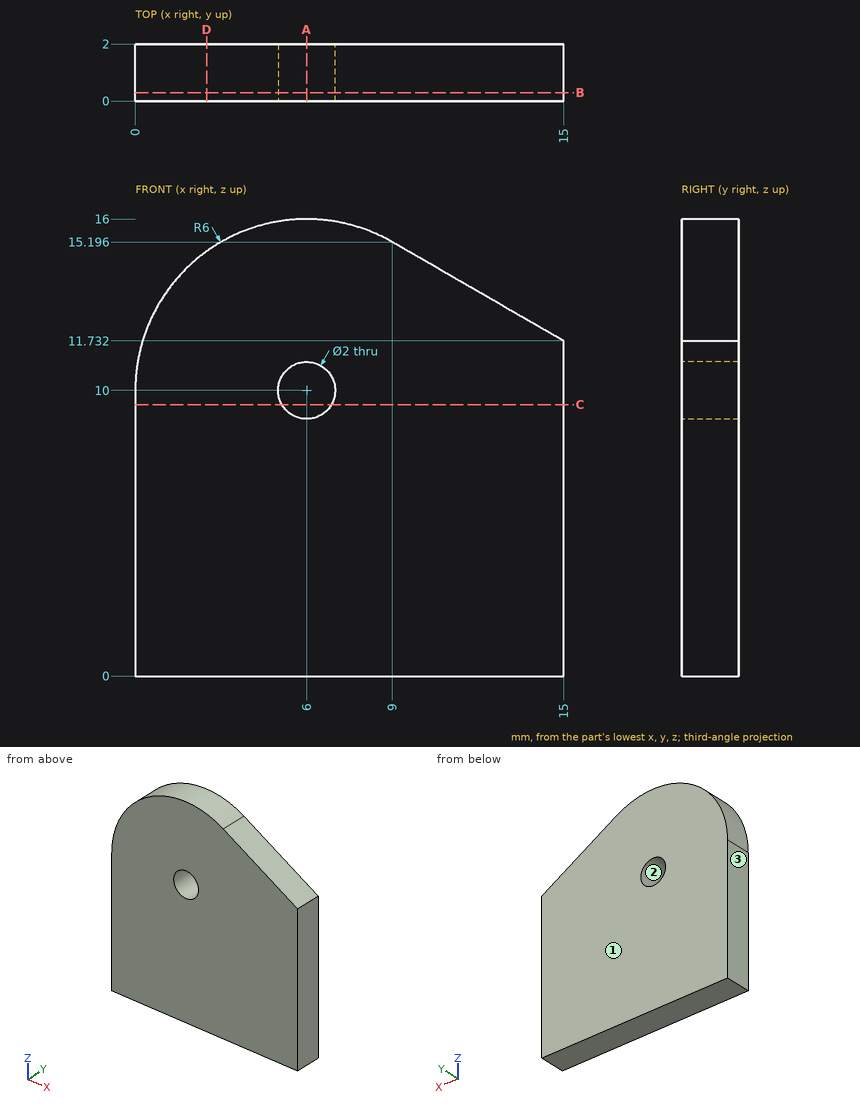
Could you check a few things on this drawing? It's one solid part, dimensions in mm from its lowest x, y, z. Coordinates: 2 decimals unless noted, no trailing zeros. Loops run counter-clockwise (first coordinate to the right, second up) from the corner with the lowest first, then second, coordinate; pieces in that order, holes last.
1. We'd pull the mould along X, two halves only. Please class the marked faces 1, 2 and 3: released by +X, released by -X, zero draft, split by the parting line, or undercut.
2. Imagine slicing it at A-A (x = 6). Please give me the cut outline in (y, z), and give its area (3 significant figures).
3. Imagine slicing it at B-B (y = 0.3). Please give me the cut outline in (x, z).
4. I need wall thicknesses on L1, parallel to Z at x = 6, y = 0.6; L2, parallel to X at y = 1.1, z = 10; L3, parallel to X at y = 1.15, z = 12 (1 decimal). Which ranges of each line are inside material? Lowest first, please.
5. Imagine slicing it at D-D (x = 2.5). Please give me the cut outline in (y, z).
6. Imagine slicing it at C-C (z = 9.5). Please give me the cut outline in (x, y).
7. For P1, Ø1.6, axis at x = 6, z = 10, coming from the +Y side, with a flat end and sliding along its axis, tell me the tip position at first contact or that it passes through.
Computed values:
1. face 1: zero draft
1. face 2: undercut
1. face 3: released by -X
2. outline: (0, 0) - (2, 0) - (2, 9) - (0, 9) - close; (0, 11) - (2, 11) - (2, 16) - (0, 16) - close
2. area: 28.0 mm2
3. outline: (0, 0) - (15, 0) - (15, 11.73) - (9, 15.2) arc R6 ccw to (0, 10) - close; hole circle Ø2 at (6, 10)
4. L1: z = 0 to 9, 11 to 16
4. L2: x = 0 to 5, 7 to 15
4. L3: x = 0.3 to 14.5
5. outline: (0, 0) - (2, 0) - (2, 14.87) - (0, 14.87) - close
6. outline: (0, 0) - (5.13, 0) - (5.13, 2) - (0, 2) - close; (6.87, 0) - (15, 0) - (15, 2) - (6.87, 2) - close
7. P1: passes through
